from build123d import *

# Parameters (mm, degrees)
SKETCH1_W           = 140
SKETCH1_H           = 207
SKETCH1_R           = 3
BOSS_EXTRUDE1_DEPTH = 10
SKETCH2_R           = 48
SKETCH2_R_2         = 40
BOSS_EXTRUDE2_DEPTH = 25
SKETCH3_R           = 20
CUT_EXTRUDE1_DEPTH  = 25
FILLET1_R           = 5
SKETCH4_R           = 30
CUT_EXTRUDE2_DEPTH  = 4
FILLET2_R           = 12


with BuildPart() as part:
    # Sketch1 → Boss-Extrude1 (new body)
    with BuildSketch(Plane.XY):
        Rectangle(SKETCH1_W, SKETCH1_H)
        with Locations((-35, 93.5)):
            Circle(SKETCH1_R, mode=Mode.SUBTRACT)
        with Locations((35, 93.5)):
            Circle(SKETCH1_R, mode=Mode.SUBTRACT)
        with Locations(Location((35, -93.5, 0), (0, 0, 180))):
            Circle(SKETCH1_R, mode=Mode.SUBTRACT)
        with Locations(Location((-35, -93.5, 0), (0, 0, 180))):
            Circle(SKETCH1_R, mode=Mode.SUBTRACT)
        with Locations((-60, -43.5)):
            Circle(SKETCH1_R, mode=Mode.SUBTRACT)
        with Locations((-60, 43.5)):
            Circle(SKETCH1_R, mode=Mode.SUBTRACT)
        with Locations(Location((60, 43.5, 0), (0, 0, 180))):
            Circle(SKETCH1_R, mode=Mode.SUBTRACT)
        with Locations(Location((60, -43.5, 0), (0, 0, 180))):
            Circle(SKETCH1_R, mode=Mode.SUBTRACT)
    extrude(amount=BOSS_EXTRUDE1_DEPTH)

    # Sketch2 → Boss-Extrude2 (add)
    with BuildSketch(Plane.XY.offset(10)):
        with Locations(Location((0, 0, 0), (0, 0, 180))):
            Circle(SKETCH2_R)
        with Locations(Location((0, 0, 0), (0, 0, 180))):
            Circle(SKETCH2_R_2, mode=Mode.SUBTRACT)
    extrude(amount=BOSS_EXTRUDE2_DEPTH)

    # Sketch3 → Cut-Extrude1 (cut)
    with BuildSketch(Plane.XY.offset(10)):
        with Locations(Location((0, 0, 0), (0, 0, 180))):
            Circle(SKETCH3_R)
    extrude(amount=-CUT_EXTRUDE1_DEPTH, mode=Mode.SUBTRACT)

    # Fillet1
    fillet1_edges = [part.edges().sort_by_distance(p)[0] for p in [
        (70, -103.5, 5),
        (-70, -103.5, 5),
        (-70, 103.5, 5),
        (70, 103.5, 5),
    ]]
    fillet(fillet1_edges, radius=FILLET1_R)

    # Sketch4 → Cut-Extrude2 (cut)
    with BuildSketch(Plane(origin=(0, 0, 0), x_dir=(-1, 0, 0), z_dir=(0, 0, -1))):
        Circle(SKETCH4_R)
    extrude(amount=-CUT_EXTRUDE2_DEPTH, mode=Mode.SUBTRACT)

    # Fillet2
    fillet2_edges = [part.edges().sort_by_distance(p)[0] for p in [
        (48, 0, 10),
    ]]
    fillet(fillet2_edges, radius=FILLET2_R)


solid = part.part
Could you check a few things on this model? Use its own coordinates, in mm. A direction names the side the tool comes from. Give positions to 0.01 mm unless a question says otherwise; leave off trailing zeros. Order: outer loops, then holes, each group sorted by start corner. A loop starts at its lowest first (then second) coordinate and runs counter-clockwise, first axis right, second up. Notation, with made-up numbers: (5.25, 7) -> (21.25, 7) arc R8 cw to (21.25, 12) -> close; hole circle Ø5 at (-15.75, 42.5). An arc over 180 degrees is marked (long way). Return JSON: item names as keys, results as strings.
1. Thinking about a two-plate mould opening in Y: for faces 1 (the cylindrical face through (-62.21, -41.47, 4.93)), 2 (the flat face through (70, -1, 5)), 3 (the flat face through (-1, 103.5, 5)), 4 (the flat face through (-1, -103.5, 5)), which applies, pulls with the +Y half, pulls with the -Y half, needs draft (parallel to the pull), parting line crosses it, or undercut?
Answer list:
{"face 1": "undercut", "face 2": "needs draft", "face 3": "pulls with the +Y half", "face 4": "pulls with the -Y half"}
2. Imagine slicing it at B-B on y = 0. List the corners of the cut face in (x, z) for me.
Answer list:
{"outline": "(-70, 0) -> (-30, 0) -> (-30, 4) -> (-20, 4) -> (-20, 10) -> (-40, 10) -> (-40, 35) -> (-48, 35) -> (-48, 22) arc R12 cw to (-60, 10) -> (-70, 10) -> close; (20, 4) -> (30, 4) -> (30, 0) -> (70, 0) -> (70, 10) -> (60, 10) arc R12 cw to (48, 22) -> (48, 35) -> (40, 35) -> (40, 10) -> (20, 10) -> close"}
3. On a 3-axis mill with a long thin cutter (end or side, diameter ignored), from which of +Z, -Z, +X, -X, +Y, -Y can I reach the whole of each face in a straight line? I mean faces 5 (the cylindrical face through (-68.57, 102, 5.07)), 6 (the cylindrical face through (29.97, 1.32, 1.97)), 7 (the cylindrical face through (39.96, -1.76, 22.32)). Say none if no direction works.
Answer list:
{"face 5": "+Z, -Z, -X, +Y", "face 6": "-Z", "face 7": "+Z"}
4. I need wall thicknesses on line 1 (Y direction, x = 0, z = 8.05); line 2 (X direction, y = -93.5, z = 2); line 3 (X direction, y = 45.5, z = 6). Which ranges of each line are inside material? Lowest first, please. Write a range as from..to.
Answer list:
{"line 1": "y = -103.5..-20, 20..103.5", "line 2": "x = -70..-38, -32..32, 38..70", "line 3": "x = -70..-62.24, -57.76..57.76, 62.24..70"}
5. Imagine slicing it at C-C on z = 27. List the corners of the cut face in (x, y) for me.
Answer list:
{"outline": "circle Ø96 at (0, 0); hole circle Ø80 at (0, 0)"}
6. For pin 1 Ø5 at (x, z) = (0, 18) entering from -Y; pin 2 Ø5 at (x, y) = (-35, 93.5) entering from -Z; pin 3 Ø6 at (y, z) = (31, 27.5) entering from -X; pin 4 Ø10 at (x, z) = (42.5, 24.5) entering from -Y, each with a flat end and sliding along its axis, tell me the tip position at first contact or that it passes through.
Answer list:
{"pin 1": "stops at y = -49.91", "pin 2": "passes through", "pin 3": "stops at x = -38.99", "pin 4": "stops at y = -29.96"}
7. Imagine slicing it at A-A on y = 93.5. List the corners of the cut face in (x, z) for me.
Answer list:
{"outline": "(-70, 0) -> (-38, 0) -> (-38, 10) -> (-70, 10) -> close; (-32, 0) -> (32, 0) -> (32, 10) -> (-32, 10) -> close; (38, 0) -> (70, 0) -> (70, 10) -> (38, 10) -> close"}
8. Imagine slicing it at D-D on y = -43.5. Give the number of separate pieces and of enclosed holes in the cut face, then the cut area to 3 significant figures.
Answer list:
{"separate pieces": "3", "enclosed holes": "0", "area": "2,420 mm2"}
